Autodesk Inventor part; units mm, degrees
ref_plane "YZ Plane" through (0, 0, 0) normal (1, 0, 0) x (0, 1, 0)
ref_plane "XZ Plane" through (0, 0, 0) normal (0, 1, 0) x (-1, 0, 0)
ref_plane "XY Plane" through (0, 0, 0) normal (0, 0, 1) x (1, 0, 0)
sketch "Skizze1" plane through (0, 0, 0) normal (0, 0, 1) x (1, 0, 0)
  line L0 (-100, 0) -> (100, 0)
  line L1 (100, 0) -> (100, 140)
  line L2 (100, 140) -> (-100, 140)
  line L3 (-100, 140) -> (-100, 0)
  point P0 (0, 0)
  dimension "d0" = 200
  dimension "d1" = 140
extrude "Extrusion1" add sketch "Skizze1" along normal blind 200
sketch "Skizze2" plane through (-100, 140, 0) normal (0, 1, 0) x (1, 0, 0)
  circle A0 centre (100, -250) radius 100
  point P0 (100, 0)
  dimension "d4" = 200
extrude "Extrusion2" cut sketch "Skizze2" against normal blind 140
sketch "Skizze3" plane through (0, 0, 0) normal (0, 0, -1) x (-1, 0, 0)
  point P0 (0, 0)
sketch "Skizze4" plane through (0, 0, 0) normal (0, 0, -1) x (-1, 0, 0)
  line L0 (15, 68) -> (-15, 68)
  line L1 (-15, 68) -> (-15, 60)
  line L2 (-15, 60) -> (15, 60)
  line L3 (15, 60) -> (15, 68)
  line L4 (-15, 76) -> (15, 76)
  line L5 (15, 76) -> (15, 84)
  line L6 (15, 84) -> (-15, 84)
  line L7 (-15, 84) -> (-15, 76)
  line L8 (-15, 92) -> (15, 92)
  line L9 (15, 92) -> (15, 100)
  line L10 (15, 100) -> (-15, 100)
  line L11 (-15, 100) -> (-15, 92)
  point P0 (0, 0)
  dimension "d7" = 30
  dimension "d8" = 8
  dimension "d9" = 30
  dimension "d10" = 8
  dimension "d11" = 8
extrude "Extrusion3" add sketch "Skizze4" along normal blind 60
sketch "Skizze5" plane through (-15, 100, 0) normal (0, 1, 0) x (1, 0, 0)
  circle A0 centre (15, 30) radius 7
  line L0 (0, 60) -> (30, 60)
  arc A1 (30, 60) -> (0, 60) centre (15, 60) ccw
  point P0 (15, 0)
  dimension "d14" = 14
  dimension "d15" = 15
extrude "Extrusion4" cut sketch "Skizze5" against normal blind 40 contours A0
properties part number "Auswurf_Rampe"
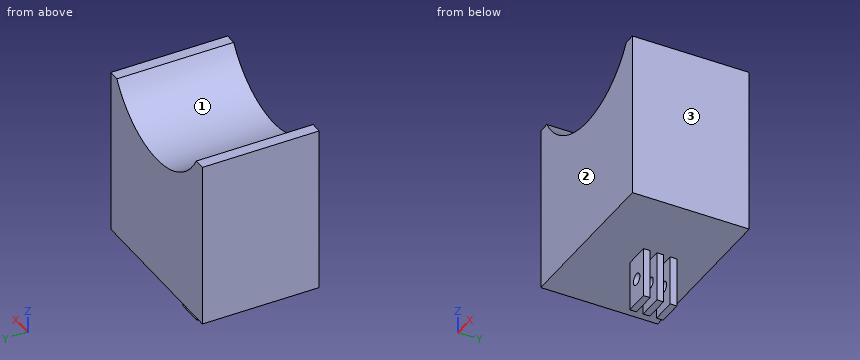
Here's how the part is built. I have some questions about the finished solid (model axes, mm). Face numbers are marked on the shaded views. Coordinates: 2 decimals unless noted, no trailing zeros. Order: outer loops, then holes, each group sorted by start corner. A loop starts at its lowest first (then second) coordinate and runs counter-clockwise, first axis right, second up.
Item 1: I'm going to push flat-ended pins straight in: pin 1 Ø2.5 at (y, z) = (94, -41.5) entering from +X; pin 2 Ø2.5 at (y, z) = (64.5, -19.5) entering from -X; pin 3 Ø12.5 at (x, z) = (0, -30) entering from -Y; pin 4 Ø24 at (x, z) = (6, -16) entering from +Y. Where does each tip first touch, or does it pass through?
Response values:
pin 1: stops at x = 15
pin 2: stops at x = -15
pin 3: passes through
pin 4: stops at y = 100
Item 2: If we section it at B-B, the plane x = 0: List the corners of the cut face in (y, z) for me.
Response values:
outline: (0, 0) - (60, 0) - (60, -23) - (68, -23) - (68, 0) - (76, 0) - (76, -23) - (84, -23) - (84, 0) - (92, 0) - (92, -23) - (100, -23) - (100, 0) - (140, 0) - (140, 150) - (0, 150) - close; (60, -60) - (68, -60) - (68, -37) - (60, -37) - close; (76, -60) - (84, -60) - (84, -37) - (76, -37) - close; (92, -60) - (100, -60) - (100, -37) - (92, -37) - close
Item 3: If we section it at C-C, the plane y = 129.5: List the corners of the cut face in (x, z) for me, then the cut area to 3 significant figures.
Response values:
outline: (-100, 0) - (100, 0) - (100, 200) - (86.6, 200) arc R100 cw to (-86.6, 200) - (-100, 200) - close
area: 33,900 mm2
Item 4: If we section it at A-A, the plane z = -30: List the corners of the cut face in (x, y) for me, then the cut area to 3 significant figures.
Response values:
outline: (-15, 60) - (-7, 60) - (-7, 68) - (-15, 68) - close; (-15, 76) - (-7, 76) - (-7, 84) - (-15, 84) - close; (-15, 92) - (-7, 92) - (-7, 100) - (-15, 100) - close; (7, 60) - (15, 60) - (15, 68) - (7, 68) - close; (7, 76) - (15, 76) - (15, 84) - (7, 84) - close; (7, 92) - (15, 92) - (15, 100) - (7, 100) - close
area: 384 mm2
Item 5: I need wall thicknesses on probe 1 along Z at (x, y) = (0, 98); probe 2 along X at (y, z) = (63.25, -30); probe 3 along Z at (x, y) = (-1.5, 121.5). Which ranges of each line are inside material? Lowest first, please.
Response values:
probe 1: z = -60 to -37, -23 to 150
probe 2: x = -15 to -7, 7 to 15
probe 3: z = 0 to 150.01
Item 6: If we section it at D-D, the plane x = 22: List the corners of the cut face in (y, z) for me, then the cut area to 3 significant figures.
Response values:
outline: (0, 0) - (140, 0) - (140, 152.45) - (0, 152.45) - close
area: 21,300 mm2
Item 7: Thinking about a two-plate mould opening in X: for the marked faces 1, 2 and 3, which applies, pulls with the +X half, pulls with the -X half, needs draft (parallel to the pull), parting line crosses it, or undercut?
Response values:
face 1: undercut
face 2: needs draft
face 3: pulls with the +X half
